```python
from build123d import *

# Parameters (mm, degrees)
BOSS_EXTRUDE2_DEPTH             = 222.249999
BOSS_EXTRUDE2_DEPTH_BACK        = 222.249999
F_1_4_0_25_DIAMETER_HOLE1_D     = 6.35
F_1_4_0_25_DIAMETER_HOLE1_DEPTH = 25.4
F_1_4_0_25_DIAMETER_HOLE1_TIP   = 1.907732465
F_1_4_0_25_DIAMETER_HOLE2_D     = 6.35
F_1_4_0_25_DIAMETER_HOLE2_DEPTH = 25.4
F_1_4_0_25_DIAMETER_HOLE2_TIP   = 1.907732465


with BuildPart() as part:
    # Sketch3 → Boss-Extrude2 (new, two sides: drawn at the far end of the back side and taken through both)
    with BuildSketch(Plane.XY.offset(-BOSS_EXTRUDE2_DEPTH_BACK)):
        Polygon((-6.35, -3.666174209), (0, -7.332348419), (6.35, -3.666174209), (6.35, 3.666174209), (0, 7.332348419), (-6.35, 3.666174209), align=None)
    extrude(amount=BOSS_EXTRUDE2_DEPTH + BOSS_EXTRUDE2_DEPTH_BACK)

    # 1/4 (0.25) Diameter Hole1
    with Locations(Plane.XY.offset(222.249999492)):
        with Locations((0, 0)):
            Hole(F_1_4_0_25_DIAMETER_HOLE1_D / 2, depth=F_1_4_0_25_DIAMETER_HOLE1_DEPTH)
            with Locations((0, 0, -(F_1_4_0_25_DIAMETER_HOLE1_DEPTH + F_1_4_0_25_DIAMETER_HOLE1_TIP / 2))):  # 118° drill point
                Cone(0, F_1_4_0_25_DIAMETER_HOLE1_D / 2, F_1_4_0_25_DIAMETER_HOLE1_TIP, mode=Mode.SUBTRACT)

    # 1/4 (0.25) Diameter Hole2
    with Locations(Plane(origin=(0, 0, -222.249999492), x_dir=(-1, 0, 0), z_dir=(0, 0, -1))):
        with Locations((0, 0)):
            Hole(F_1_4_0_25_DIAMETER_HOLE2_D / 2, depth=F_1_4_0_25_DIAMETER_HOLE2_DEPTH)
            with Locations((0, 0, -(F_1_4_0_25_DIAMETER_HOLE2_DEPTH + F_1_4_0_25_DIAMETER_HOLE2_TIP / 2))):  # 118° drill point
                Cone(0, F_1_4_0_25_DIAMETER_HOLE2_D / 2, F_1_4_0_25_DIAMETER_HOLE2_TIP, mode=Mode.SUBTRACT)


solid = part.part
```
Could you check a few things on this model? Use its own coordinates, in mm. Give positions to 0.01 mm unless a question says otherwise; leave off trailing zeros. Write each loop counter-clockwise with the first axis right and the second up, starting at its lowest first coordinate (ties: lowest second). Pieces come first, ordered by that corner, then holes. Notation, with made-up numbers: (50.25, 7.5) - (66.25, 7.5) arc R36 cw to (66.25, 45.5) - close; hole circle Ø6 at (-35, 69.5). An arc over 180 degrees is marked (long way). One line per item, written item: value. Start each with the question number.
Item 1: Please list where these lines run through material, in increasing order: line 1 (Y direction, x = 0, z = 207.5) (3 decimals); line 2 (X direction, y = 0, z = -211.5) (3 decimals); line 3 (Z direction, x = 0.75, y = -1). Write a range as from..to.
Item 2: I'm going to push flat-ended pins straight in: pin 1 (4 mm diameter, centred on x = 1.5, z = -71, fed in from -Y); pin 2 (2 mm diameter, centred on y = -6, z = -70, fed in from -X); pin 3 (5 mm diameter, centred on x = 0, y = 0, fed in from +Z). Where does each tip first touch, or does it pass through?
Item 3: Imagine slicing it at A-A, the plane z = -131. List the corners of the cut face in (x, y) for me.
Geometry says:
1. line 1: -7.332..-3.175, 3.175..7.332
1. line 2: -6.35..-3.175, 3.175..6.35
1. line 3: -195.69..195.69
2. pin 1: y = -7.33
2. pin 2: x = -4.04
2. pin 3: z = 196.44
3. outline: (-6.35, -3.67) - (0, -7.33) - (6.35, -3.67) - (6.35, 3.67) - (0, 7.33) - (-6.35, 3.67) - close
